```python
from build123d import *

# Parameters (mm, degrees)
SKETCH1_W                   = 300
SKETCH1_H                   = 200
SKETCH1_W_2                 = 30
SKETCH1_H_2                 = 40
BOSS_EXTRUDE1_DEPTH         = 6.35
TAP_DRILL_FOR_M4X0_7_TAP1_D = 3.3
M3_CLEARANCE_HOLE1_D        = 3.2
M5_CLEARANCE_HOLE1_D        = 5.3
FILLET1_R                   = 1


with BuildPart() as part:
    # Sketch1 → Boss-Extrude1 (new body)
    with BuildSketch(Plane(origin=(0, 0, 0), x_dir=(1, 0, 0), z_dir=(0, 1, 0))):
        Rectangle(SKETCH1_W, SKETCH1_H)
        with Locations((0, -40)):
            Rectangle(SKETCH1_W_2, SKETCH1_H_2, mode=Mode.SUBTRACT)
    extrude(amount=-BOSS_EXTRUDE1_DEPTH)

    # Tap Drill for M4x0.7 Tap1 (through all)
    with Locations(Plane(origin=(-112.5, 0, -32.5), x_dir=(0, 0, 1), z_dir=(0, 1, 0))):
        with Locations((0, 0), (30, 0), (0, 225), (30, 225)):
            Hole(TAP_DRILL_FOR_M4X0_7_TAP1_D / 2)

    # M3 Clearance Hole1 (through all)
    with Locations(Plane(origin=(-59, 0, 30), x_dir=(0, 0, 1), z_dir=(0, 1, 0))):
        with Locations((0, 0), (0, 34), (40, 0), (40, 34), (0, 84), (0, 118), (40, 84), (40, 118)):
            Hole(M3_CLEARANCE_HOLE1_D / 2)

    # M5 Clearance Hole1 (through all)
    with Locations(Plane(origin=(-140, 0, -90), x_dir=(0, 0, 1), z_dir=(0, 1, 0))):
        with Locations((0, 0), (0, 140), (0, 280), (180, 280), (180, 140), (180, 0), (90, 140)):
            Hole(M5_CLEARANCE_HOLE1_D / 2)

    # Fillet1
    fillet1_edges = [part.edges().sort_by_distance(p)[0] for p in [
        (15, -3.175, 20),
        (15, -3.175, 60),
        (-15, -3.175, 60),
        (-15, -3.175, 20),
    ]]
    fillet(fillet1_edges, radius=FILLET1_R)


solid = part.part
```
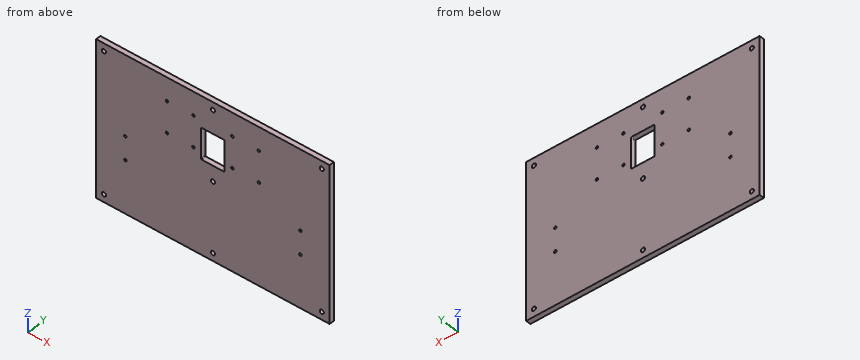
Here's how the part is built. I have some questions about the finished solid (model axes, mm). Give positions to 0.01 mm unless a question says otherwise; leave off trailing zeros. Order: outer loops, then holes, each group sorted by start corner. A loop starts at its lowest first (then second) coordinate and runs counter-clockwise, first axis right, second up. Notation, with made-up numbers: (-26.5, -9) - (25.5, -9) arc R24 cw to (25.5, 8) - close; hole circle Ø1 at (-22, -39). An arc over 180 degrees is marked (long way). Answer as a JSON object with one key per item and string values. Group by question number.
Item 1: If we section it at B-B on y = -1.25: Give the number of separate pieces and of enclosed holes in the cut face, and give its area (3 significant figures).
Item 2: Please list where these lines run through material, in increasing order: probe 1 along X at (y, z) = (-4, 70); probe 2 along X at (y, z) = (-1.75, -90); probe 3 along X at (y, z) = (-2.5, -32.5).
Item 3: If we section it at A-A on z = 42: Please give me the cut outline in (x, y).
Result set:
{
 "1": {"separate pieces": "1", "enclosed holes": "20", "area": "58,500 mm²"},
 "2": {"probe 1": "-150 to -60.6, -57.4 to -26.6, -23.4 to 23.4, 26.6 to 57.4, 60.6 to 150", "probe 2": "-150 to -142.65, -137.35 to -2.65, 2.65 to 137.35, 142.65 to 150", "probe 3": "-150 to -114.15, -110.85 to 110.85, 114.15 to 150"},
 "3": {"outline": "(-150, -6.35) - (-15, -6.35) - (-15, 0) - (-150, 0) - close; (15, -6.35) - (150, -6.35) - (150, 0) - (15, 0) - close"}
}
